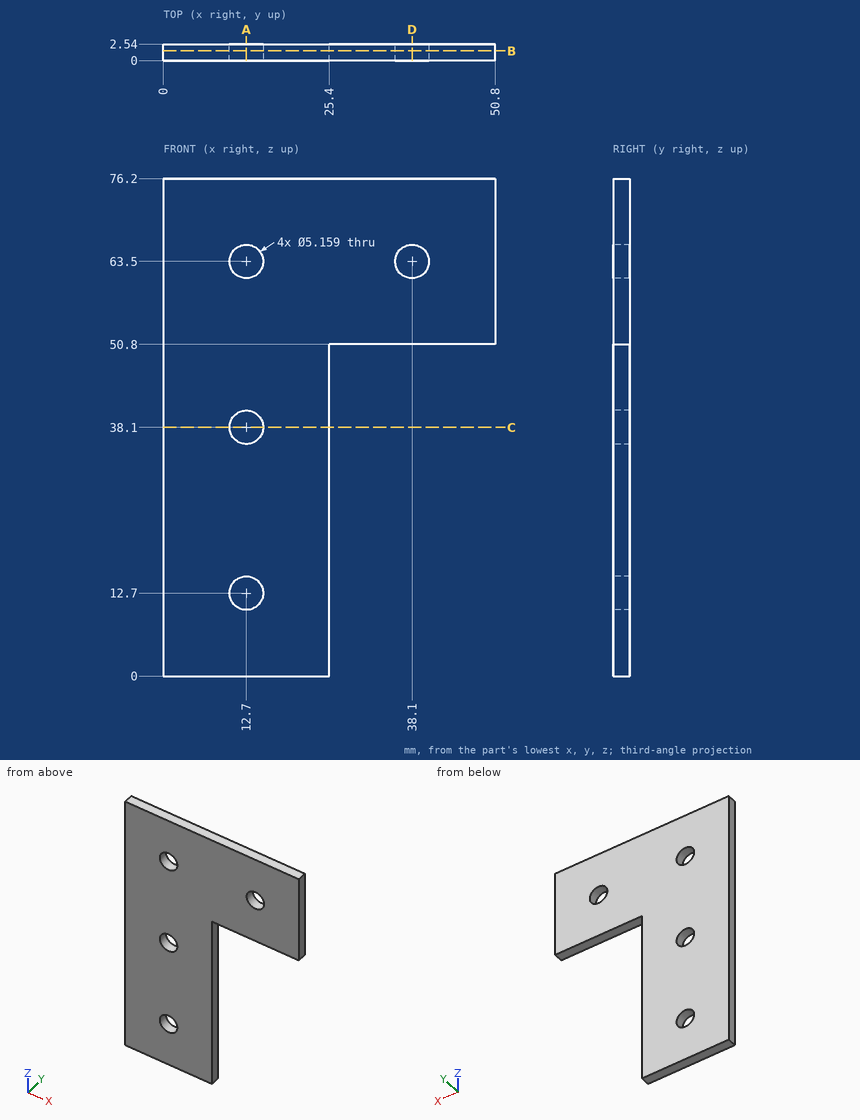
Could you check a few things on this drawing? It's one solid part, dimensions in mm from its lowest x, y, z. Give positions to 0.01 mm unless a question says otherwise; leave off trailing zeros. Loops run counter-clockwise (first coordinate to the right, second up) from the corner with the lowest first, then second, coordinate; pieces in that order, holes last. Notation, with made-up numbers: M -34,-36 L 20,-36 A25 ccw 20,0 Z; hole C 34,-32 d6. An arc over 180 degrees is marked long. Answer as a JSON object with one key per item and string values.
Q1. Suppose I cut it at C-C, the plane z = 38.1. List the corners of the cut face in (x, y) for me.
Values found:
{"outline": "M 0,0 L 10.12,0 L 10.12,2.54 L 0,2.54 Z; M 15.28,0 L 25.4,0 L 25.4,2.54 L 15.28,2.54 Z"}
Q2. Suppose I cut it at D-D, the plane x = 38.1. List the corners of the cut face in (y, z) for me.
Values found:
{"outline": "M 0,50.8 L 2.54,50.8 L 2.54,60.92 L 0,60.92 Z; M 0,66.08 L 2.54,66.08 L 2.54,76.2 L 0,76.2 Z"}
Q3. Suppose I cut it at A-A, the plane x = 12.7. List the corners of the cut face in (y, z) for me, plus the area to 3 significant figures.
Values found:
{"outline": "M 0,0 L 2.54,0 L 2.54,10.12 L 0,10.12 Z; M 0,15.28 L 2.54,15.28 L 2.54,35.52 L 0,35.52 Z; M 0,40.68 L 2.54,40.68 L 2.54,60.92 L 0,60.92 Z; M 0,66.08 L 2.54,66.08 L 2.54,76.2 L 0,76.2 Z", "area": "154 mm²"}
Q4. If I drill on probe 1 along Z at (x, y) = (12.7, 2); probe 2 along X at (y, z) = (2.1, 26); probe 3 along Z at (x, y) = (36, 1.15), over which ranges is the centre line in solid material (lowest first)? Write a range as [from, to].
Values found:
{"probe 1": "z = [0, 10.12], [15.28, 35.52], [40.68, 60.92], [66.08, 76.2]", "probe 2": "x = [0, 25.4]", "probe 3": "z = [50.8, 62], [65, 76.2]"}
Q5. Suppose I cut it at B-B, the plane y = 1.5. List the corners of the cut face in (x, z) for me.
Values found:
{"outline": "M 0,0 L 25.4,0 L 25.4,50.8 L 50.8,50.8 L 50.8,76.2 L 0,76.2 Z; hole C 12.7,12.7 d5.16; hole C 12.7,38.1 d5.16; hole C 12.7,63.5 d5.16; hole C 38.1,63.5 d5.16"}
Q6. For P1, Ø0.8, axis at y = 1, z = 29, coming from the +X side; P2, Ø1.3, axis at x = 43.5, y = 1.5, coming from the -Z side, each with a flat end and sliding along its axis, tell me the tip position at first contact or that it passes through.
Values found:
{"P1": "stops at x = 25.4", "P2": "stops at z = 50.8"}
